Verification items for this drawing (mm, ordinates from the low corner). Coordinates: 2 decimals unless noted, no trailing zeros. Loops run counter-clockwise (first coordinate to the right, second up) from the corner with the lowest first, then second, coordinate; pieces in that order, holes last. Notation, with made-up numbers: M 74,60.5 L 96,60.5 A29 ccw 96,91.5 Z; hole C -22.5,-11 d3. An arc over 180 degrees is marked long. Use CSV: the item, a comma, the result in double quotes.
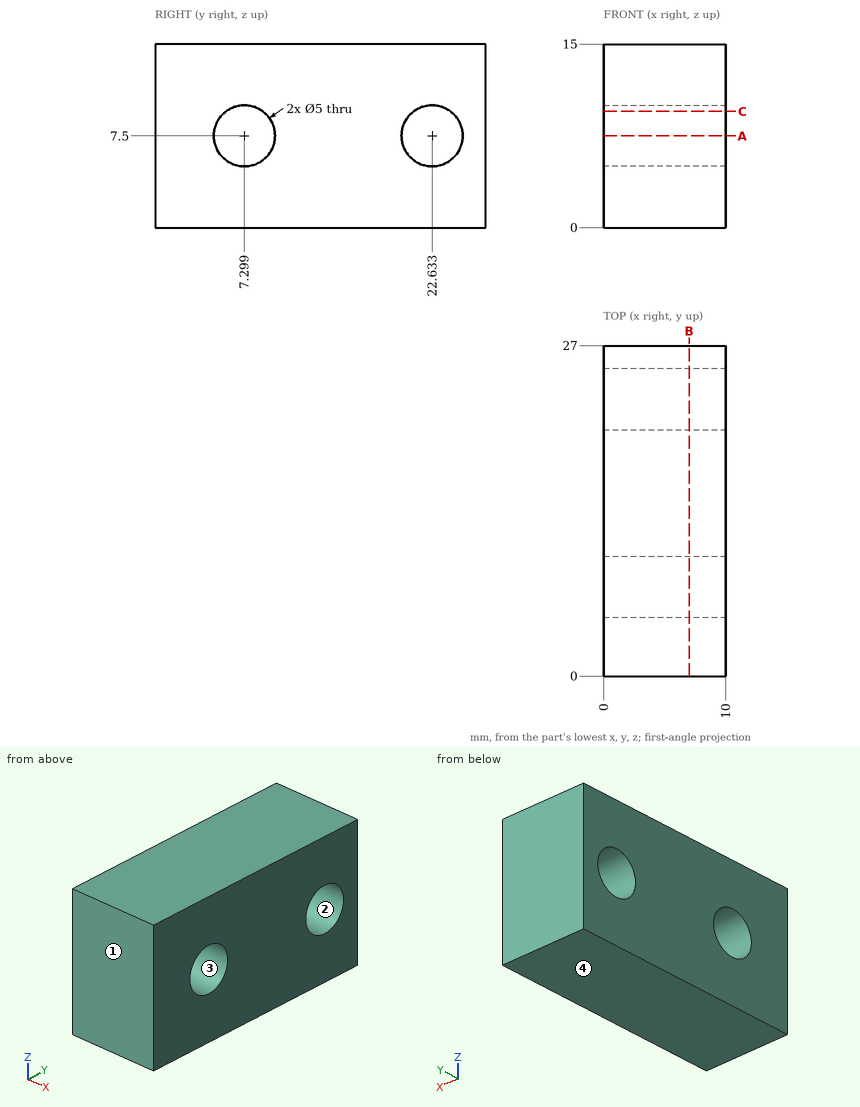
1. Release check for a two-part mould opening along Y. For the marked faces 1, 2, 3 and 4 record: +Y half, -Y half, draft (parallel to the pull), parting line (faces both ways), or undercut.
The answers:
face 1,"-Y half"
face 2,"undercut"
face 3,"undercut"
face 4,"draft"
2. Section check A-A, the plane z = 7.5. Record the cut outline in (x, y).
The answers:
outline,"M 0,0 L 10,0 L 10,4.8 L 0,4.8 Z; M 0,9.8 L 10,9.8 L 10,20.13 L 0,20.13 Z; M 0,25.13 L 10,25.13 L 10,27 L 0,27 Z"
3. Thickness scan on line 1 (Y direction, x = 3, z = 7.5); line 2 (Y direction, x = 2.75, z = 7); line 3 (Z direction, x = 6, y = 6.25). Record the ranges inside material, lowest first. Write a range as [from, to].
The answers:
line 1,"[0, 4.8], [9.8, 20.13], [25.13, 27]"
line 2,"[0, 4.85], [9.75, 20.18], [25.08, 27]"
line 3,"[0, 5.23], [9.77, 15]"
4. Section check C-C, the plane z = 9.5. Record the cut outline in (x, y), plus the area to 3 significant figures.
The answers:
outline,"M 0,0 L 10,0 L 10,5.8 L 0,5.8 Z; M 0,8.8 L 10,8.8 L 10,21.13 L 0,21.13 Z; M 0,24.13 L 10,24.13 L 10,27 L 0,27 Z"
area,"210 mm^2"
5. Section check B-B, the plane x = 7. Record the cut outline in (y, z).
The answers:
outline,"M 0,0 L 27,0 L 27,15 L 0,15 Z; hole C 7.3,7.5 d5; hole C 22.63,7.5 d5"
